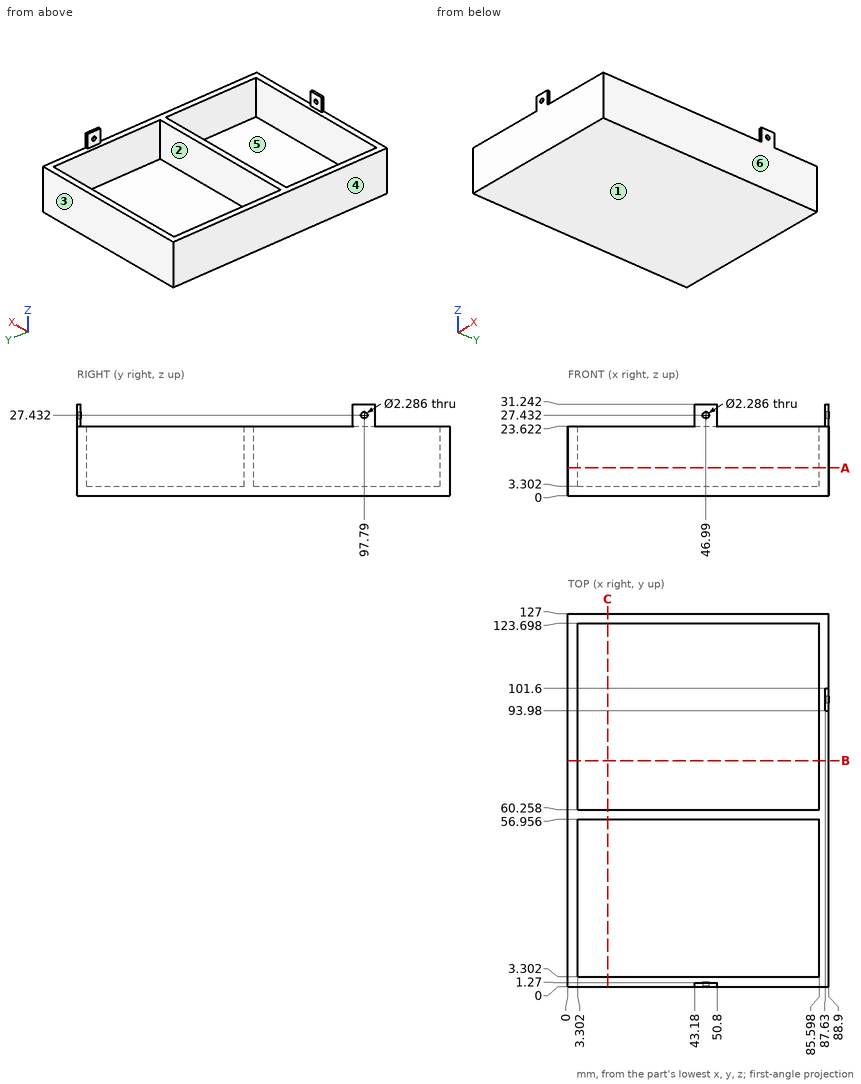
Input: dimensioned drawing with shaded views. Units: mm. Origin: part minimum x, y, z. A direction names the side the tool comes from. Round coordinates to 2 decimals unless told otherwise and drop trailing zeros. Loops run counter-clockwise (first coordinate to the right, second up) from the corner with the lowest first, then second, coordinate; pieces in that order, holes last. Notation, with made-up numbers: M 14,-6 L 44,-6 A11 ccw 44,0 Z; hole C 60,38.25 d2. An arc over 180 degrees is marked long. One line per question, with ' | ' between items.
(1) Cut plane C-C on x = 13.5. Return the cut outline in (y, z), plus the area to 3 significant figures.
Check result:
outline: M 0,0 L 127,0 L 127,23.62 L 123.7,23.62 L 123.7,3.3 L 60.26,3.3 L 60.26,23.62 L 56.96,23.62 L 56.96,3.3 L 3.3,3.3 L 3.3,23.62 L 0,23.62 Z | area: 621 mm2
(2) Cut plane B-B on y = 77. Return the cut outline in (x, z).
Check result:
outline: M 0,0 L 88.9,0 L 88.9,23.62 L 85.6,23.62 L 85.6,3.3 L 3.3,3.3 L 3.3,23.62 L 0,23.62 Z
(3) Material intervals for line 1 along Y through (x, z) = (83, 18.5); line 2 along X through (y, z) = (63, 16); line 3 along Z through (x, y) = (88.1, 97.79) (3 decimals), sorted ascending. Write a range as from..to.
Check result:
line 1: y = 0..3.3, 56.96..60.26, 123.7..127 | line 2: x = 0..3.3, 85.6..88.9 | line 3: z = 0..26.289, 28.575..31.242
(4) Pull-direction query (X, two-part tool) for the marked faces 3, 4, 5 and 6; classes: +X half, -X half, draft (parallel to the pull), parting line (faces both ways), or undercut.
Check result:
face 3: draft | face 4: -X half | face 5: undercut | face 6: +X half
(5) Cut plane A-A on z = 9.5. Return the cut outline in (x, y), plus the area to 3 significant figures.
Check result:
outline: M 0,0 L 88.9,0 L 88.9,127 L 0,127 Z; hole M 3.3,3.3 L 85.6,3.3 L 85.6,56.96 L 3.3,56.96 Z; hole M 3.3,60.26 L 85.6,60.26 L 85.6,123.7 L 3.3,123.7 Z | area: 1,650 mm2
(6) Access query for the marked faces 1 and 2. Directions: +Z, -Z, +X, -X, +Y, -Y. A direction counts if a zero-diameter tool reaches every point of the face in a straight line with its end or side. Return the directions, or none.
Check result:
face 1: -Z, +X, -X, +Y, -Y | face 2: +Z
(7) Contact query for flat-ended pins moving along their axis: P1, Ø8, axis at x = 48.5, z = 28, coming from the +Y side; P2, Ø1, axis at x = 88, z = 26.5, coming from the -Y side; P3, Ø12, axis at x = 64.5, y = 28, coming from the +Z side. Output: stop coordinate, or through.
Check result:
P1: stops at y = 1.27 | P2: stops at y = 93.98 | P3: stops at z = 3.3
